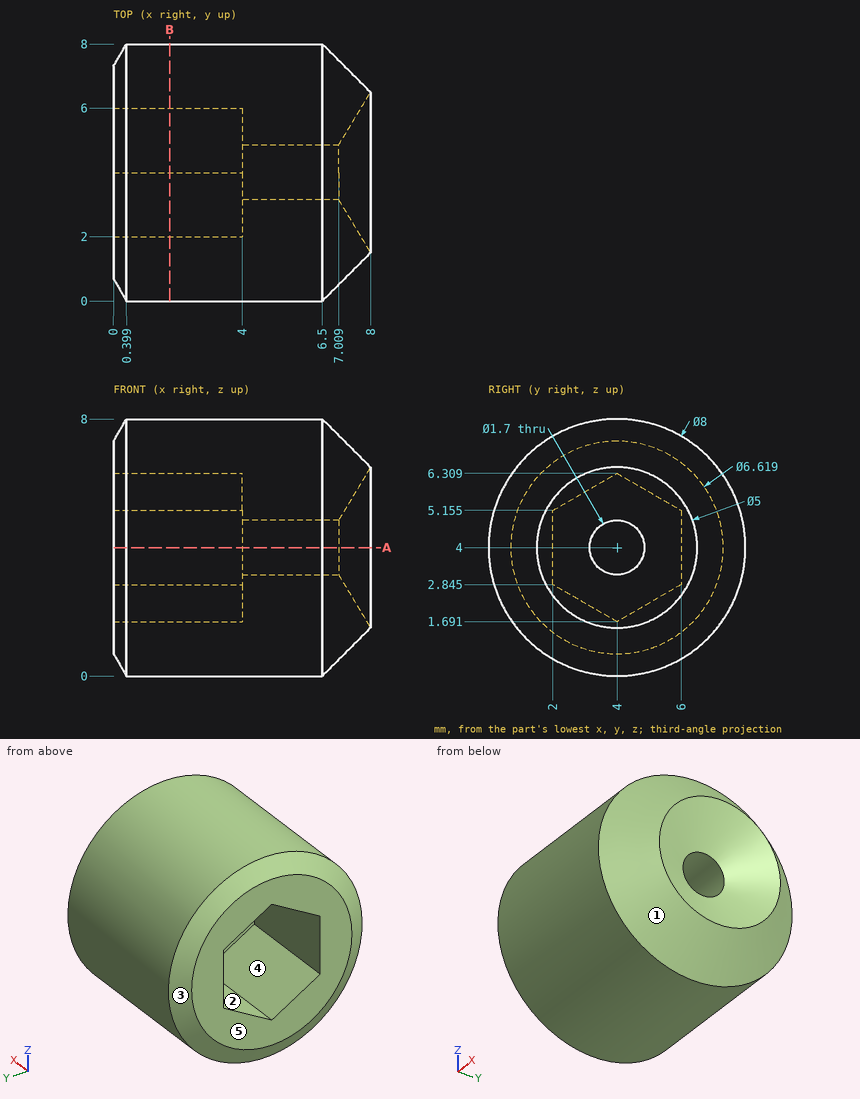
Study the drawing (mm; zero at the part's minimum x, y, z) and answer. A direction names the side the tool comes from. Round coordinates to 2 decimals unless told otherwise and drop trailing zeros. Write each loop counter-clockwise with the first axis right and the second up, starting at its lowest first coordinate (ties: lowest second). Pieces come first, ordered by that corner, then holes. Notation, with made-up numbers: (28.25, 81.5) -> (71.25, 81.5) arc R28 ccw to (71.25, 111.5) -> close; hole circle Ø7 at (-37.75, 75). An arc over 180 degrees is marked (long way). Use CSV: the item, a comma, the result in double quotes. Start each with the question number.
(1) The mould has two halves that part along Z. Classify the marked faces 3, 4 and 5: released by +Z, released by -Z, zero draft, split by the parting line, or undercut.
(2) Consider L1, parallel to Z at x = 5.6, y = 4; L2, parallel to Z at x = 1.75, y = 3.75 (1 decimal). Determine where each line is inside the solid, lowest interval first. Write a range as from..to.
(3) Which of the six approach directions +Z, -Z, +X, -X, +Y, -Y give full straight-line access (tool end or side, diameter ignored) to the marked faces 1 and 2?
(4) Section B-B on x = 1.75 is taken. Give the vertices of the cut face in (y, z) (1 decimal).
(5) Each of these flat-tipped pins is pushed along its axis until it touches: pin 1 (4 mm diameter, centred on y = 2.5, z = 1, fed in from -X); pin 2 (2 mm diameter, centred on y = 4, z = 4, fed in from -X). Where does it stop, or does it pass through?
(6) Section A-A on z = 4 is taken. Give the vertices of the cut face in (x, y).
A:
1,face 3,"split by the parting line"
1,face 4,"undercut"
1,face 5,"zero draft"
2,L1,"z = 0..3.15, 4.85..8"
2,L2,"z = 0..1.8, 6.2..8"
3,face 1,"+X"
3,face 2,"-X"
4,outline,"circle Ø8 at (4, 4); hole (2, 2.8) -> (4, 1.7) -> (6, 2.8) -> (6, 5.2) -> (4, 6.3) -> (2, 5.2) -> close"
5,pin 1,"stops at x = 0"
5,pin 2,"stops at x = 4"
6,outline,"(0, 0.69) -> (0.4, 0) -> (6.5, 0) -> (8, 1.5) -> (7.01, 3.15) -> (4, 3.15) -> (4, 2) -> (0, 2) -> close; (0, 6) -> (4, 6) -> (4, 4.85) -> (7.01, 4.85) -> (8, 6.5) -> (6.5, 8) -> (0.4, 8) -> (0, 7.31) -> close"
